```python
from build123d import *

# Parameters (mm, degrees)
EXTRUDE_THIN1_DEPTH = 127
FILLET1_R           = 0.889


with BuildPart() as part:
    # Sketch1 → Extrude-Thin1 (new body)
    with BuildSketch(Plane.XY):
        with BuildLine():
            Line((0, 14.2875), (0.396875, 7.9375))
            Line((0.396875, 7.9375), (11.811, 7.9375))
            Line((11.811, 7.9375), (11.811, 5.55625))
            Line((11.811, 5.55625), (9.42975, 5.55625))
            Line((9.42975, 5.55625), (9.42975, 3.96875))
            ThreePointArc((9.42975, 3.96875), (7.038283045, 3.743245435), (5.112942469, 2.306920202))
            ThreePointArc((5.112942469, 2.306920202), (2.845206289, 0.513522178), (0, 0))
            Line((0, 0), (0.396875, 2.778125))
            Line((0.396875, 2.778125), (1.2769401, 2.652401414))
            Line((1.2769401, 2.652401414), (1.028787976, 0.915336544))
            ThreePointArc((1.028787976, 0.915336544), (2.912071238, 1.54452561), (4.408676393, 2.849442363))
            ThreePointArc((4.408676393, 2.849442363), (6.237754348, 4.359868554), (8.54075, 4.928308939))
            Line((8.54075, 4.928308939), (8.54075, 6.44525))
            Line((8.54075, 6.44525), (10.922, 6.44525))
            Line((10.922, 6.44525), (10.922, 7.0485))
            Line((10.922, 7.0485), (-0.438297136, 7.0485))
            Line((-0.438297136, 7.0485), (-0.887268742, 14.232045704))
            Line((-0.887268742, 14.232045704), (0, 14.2875))
        make_face()
    extrude(amount=-EXTRUDE_THIN1_DEPTH)

    # Fillet1
    fillet1_edges = [part.edges().sort_by_distance(p)[0] for p in [
        (8.54075, 6.44525, -63.5),
        (-0.438297136, 7.0485, -63.5),
        (11.811, 7.9375, -63.5),
        (11.811, 5.55625, -63.5),
        (9.42975, 3.96875, -63.5),
        (0, 0, -63.5),
    ]]
    fillet(fillet1_edges, radius=FILLET1_R)


solid = part.part
```
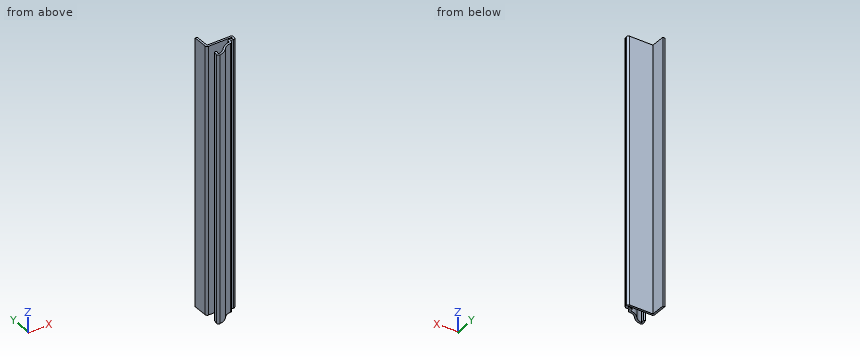
Geometry check sheet. Reference: the model listing, model coordinates, mm. Coordinates: 2 decimals unless noted, no trailing zeros. Write each loop counter-clockwise with the first axis right and the second up, starting at its lowest first coordinate (ties: lowest second). Pieces come first, ordered by that corner, then holes. Notation, with made-up numbers: M -25.75,-27 L 12.25,-27 A20 ccw 12.25,-16 Z; hole C -7.75,-1 d4. An arc over 180 degrees is marked long. Use one line per item in the form item = value. Start each with the question number.
1) Section check B-B on x = 2.75. Enter the section's corners in (y, z), and give its area (3 significant figures).
2) Section check D-D on y = 11.5. Enter the section's corners in (x, z), and give its area (3 significant figures).
3) Go/stop test with flat-tipped pins: pin 1 Ø1 at (x, z) = (5.5, -113.5) entering from +Y; pin 2 Ø5.5 at (x, z) = (4.5, -65) entering from -Y; pin 3 Ø2 at (x, y) = (1.5, 5.5) entering from +Z; pin 4 Ø1.6 at (x, z) = (10, -41.5) entering from -Y. Record where each tip stops, or that it passes through.
4) Section check A-A on z = -77.5. Enter the section's corners in (x, y), and give its area (3 significant figures).
5) Thickness scan on probe 1 along Y at (x, z) = (10.75, -108.5); probe 2 along Y at (x, z) = (1.75, -28); probe 3 along X at (y, z) = (2, -31). Record the ranges inside material, lowest first. Write a range as from..to.
6) Section check C-C on x = 7.5. Enter the section's corners in (y, z).
Responses:
q1.outline = M 0.47,-127 L 1.46,-127 L 1.46,0 L 0.47,0 Z; M 7.05,-127 L 7.94,-127 L 7.94,0 L 7.05,0 Z
q1.area = 238 mm2
q2.outline = M -0.72,-127 L 0.17,-127 L 0.17,0 L -0.72,0 Z
q2.area = 113 mm2
q3.pin_1 = 7.94
q3.pin_2 = 0.14
q3.pin_3 = through
q3.pin_4 = 4.33
q4.outline = M -0.89,14.23 L -0.49,7.88 A0.89 ccw 0.4,7.05 L 10.92,7.05 L 10.92,6.45 L 9.43,6.45 A0.89 ccw 8.54,5.56 L 8.54,4.93 A5.34 ccw 4.41,2.85 A5.06 cw 1.03,0.92 L 1.28,2.65 L 0.4,2.78 L 0.15,1.04 A0.89 ccw 1.14,0.03 A5.95 ccw 5.11,2.31 A4.45 cw 8.56,4.04 A0.89 ccw 9.43,4.93 L 9.43,5.56 L 10.92,5.56 A0.89 ccw 11.81,6.45 L 11.81,7.05 A0.89 ccw 10.92,7.94 L 0.4,7.94 L 0,14.29 Z
q4.area = 30.6 mm2
q5.probe_1 = 5.56..6.45, 7.05..7.94
q5.probe_2 = 0.14..1.06, 7.05..7.94
q5.probe_3 = 0.29..1.18, 3.58..4.86
q6.outline = M 3.89,-127 L 4.81,-127 L 4.81,0 L 3.89,0 Z; M 7.05,-127 L 7.94,-127 L 7.94,0 L 7.05,0 Z
